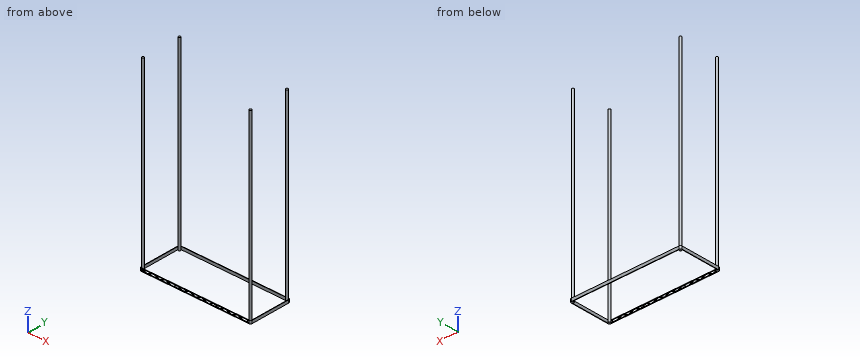
```python
from build123d import *

# Parameters (mm, degrees)
F1_DEPTH = 31
F2_R     = 12.75
F3_DEPTH = 2000
F5_DEPTH = 25


# Not quite as in the source:
# - ends of sketch curves that miss each other by under 0.0002 mm in the source are joined


with BuildPart() as f1:
    # F0 (on Top) → F1 (new body)
    with BuildSketch(Plane.XY):
        with BuildLine():
            Line((-4.9999998882, 442.5), (-4.9999998882, 12.5))
            ThreePointArc((-4.9999998882, 12.5), (0.1256313292, 0.1256313292), (12.5, -5))
            Line((12.5, -5), (1187.5, -5))
            ThreePointArc((1187.5, -5), (1199.8743686708, 0.1256313292), (1205, 12.5))
            Line((1205, 12.5), (1205, 442.5))
            ThreePointArc((1205, 442.5), (1199.8743686708, 454.8743686708), (1187.5, 460))
            Line((1187.5, 460), (12.5, 460.0000083447))
            ThreePointArc((12.5, 460.0000083447), (0.1256313292, 454.8743686708), (-4.9999998882, 442.5))
        make_face()
        with BuildLine():
            Line((1187.5, 0), (12.5, 0))
            ThreePointArc((12.5, 0), (3.6611652352, 3.6611652352), (0, 12.5))
            Line((0, 12.5), (0, 442.5))
            ThreePointArc((0, 442.5), (3.6611652352, 451.3388347648), (12.5, 455))
            Line((12.5, 455), (1187.5, 455))
            ThreePointArc((1187.5, 455), (1196.3388347648, 451.3388347648), (1200, 442.5))
            Line((1200, 442.5), (1200, 12.5))
            ThreePointArc((1200, 12.5), (1196.3388347648, 3.6611652352), (1187.5, 0))
        make_face(mode=Mode.SUBTRACT)
    extrude(amount=F1_DEPTH)

    # F2 (on Top) → F3 (join)
    with BuildSketch(Plane.XY):
        with Locations((12.7221517224, 12.6146673983)):
            Circle(F2_R)
        with Locations((12.7221517224, 442.3853326017)):
            Circle(F2_R)
        with Locations((1187.2778482776, 442.3853326017)):
            Circle(F2_R)
        with Locations((1187.2778482776, 12.6146673983)):
            Circle(F2_R)
    extrude(amount=F3_DEPTH)

    # F4 (on Front) → F5 (cut)
    with BuildSketch(Plane.XZ):
        Polygon((1187.5, 26.9953021277), (1128.762, 4), (1187.5, 4), align=None)
        Polygon((1066.012, 27), (1124.762, 4), (1183.512, 27), align=None)
        Polygon((1056.323, 27), (997.573, 4), (1120.762, 4), (1062.012, 27), align=None)
        Polygon((934.823, 27), (993.573, 4), (1052.323, 27), align=None)
        Polygon((925.134, 27), (866.384, 4), (989.573, 4), (930.823, 27), align=None)
        Polygon((803.634, 27), (862.384, 4), (921.134, 27), align=None)
        Polygon((793.945, 27), (735.195, 4), (858.384, 4), (799.634, 27), align=None)
        Polygon((672.445, 27), (731.195, 4), (789.945, 27), align=None)
        Polygon((662.756, 27), (604.006, 4), (727.195, 4), (668.445, 27), align=None)
        Polygon((541.256, 27), (600.006, 4), (658.756, 27), align=None)
        Polygon((531.567, 27), (472.817, 4), (596.006, 4), (537.256, 27), align=None)
        Polygon((410.067, 27), (468.817, 4), (527.567, 27), align=None)
        Polygon((400.378, 27), (341.628, 4), (464.817, 4), (406.067, 27), align=None)
        Polygon((278.878, 27), (337.628, 4), (396.378, 27), align=None)
        Polygon((269.189, 27), (210.439, 4), (333.628, 4), (274.878, 27), align=None)
        Polygon((265.189, 27), (147.689, 27), (206.439, 4), align=None)
        Polygon((143.689, 27), (138, 27), (79.25, 4), (202.439, 4), align=None)
        Polygon((134, 27), (16.5, 27), (75.25, 4), align=None)
        Polygon((71.25, 4), (12.5, 27), (12.5, 4), align=None)
    extrude(amount=F5_DEPTH, mode=Mode.SUBTRACT)


solid = f1.part
```
Here's how the part is built. I have some questions about the finished solid (model axes, mm). Coordinates: 2 decimals unless noted, no trailing zeros. Order: outer loops, then holes, each group sorted by start corner. A loop starts at its lowest first (then second) coordinate and runs counter-clockwise, first axis right, second up.
1) Imagine slicing it at A-A on y = 201. List the corners of the cut face in (x, z) for me.
2) Imagine slicing it at C-C on z = 1323.5. List the corners of the cut face in (x, y) for me.
3) Will these pins go through, and if not, where does the flat tip stop? pin 1 (2.5 mm diameter, centred on x = 1075, y = -2.5, fed in from +Z); pin 2 (5.5 mm diameter, centred on y = -1.5, z = 14.5, fed in from +X).
4) Imagine slicing it at B-B on x = 625.5. List the corners of the cut face in (y, z) for me, and give its area (3 significant figures).
Response values:
1. outline: (-5, 0) - (0, 0) - (0, 31) - (-5, 31) - close; (1200, 0) - (1205, 0) - (1205, 31) - (1200, 31) - close
2. outline: circle Ø25.5 at (12.72, 12.61); circle Ø25.5 at (12.72, 442.39); circle Ø25.5 at (1187.28, 12.61); circle Ø25.5 at (1187.28, 442.39)
3. pin 1: stops at z = 31
3. pin 2: stops at x = 1200.9
4. outline: (-5, 0) - (0, 0) - (0, 4) - (-5, 4) - close; (-5, 12.41) - (0, 12.41) - (0, 13.98) - (-5, 13.98) - close; (-5, 27) - (0, 27) - (0, 31) - (-5, 31) - close; (455, 0) - (460, 0) - (460, 31) - (455, 31) - close
4. area: 203 mm2
